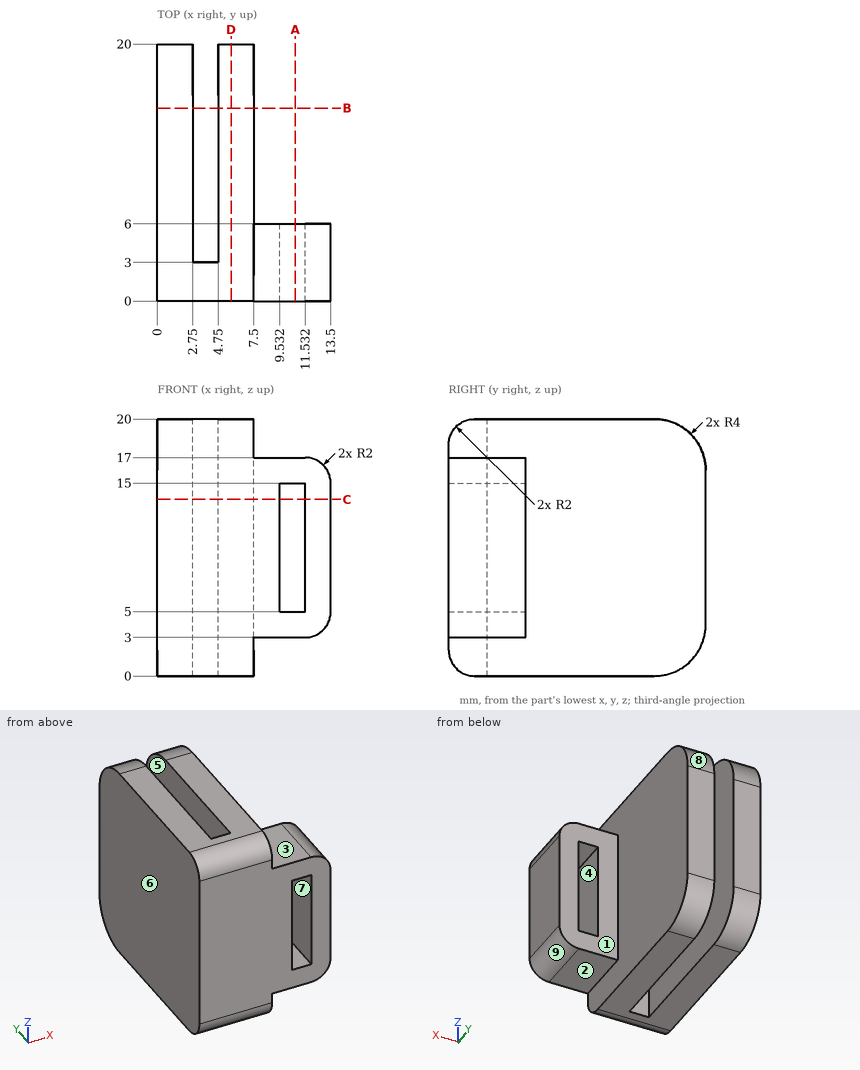
Verification items for this drawing (mm, ordinates from the low corner). A direction names the side the tool comes from. Give positions to 0.01 mm unless a question says otherwise; leave off trailing zeros. Write each loop counter-clockwise with the first axis right and the second up, starting at its lowest first coordinate (ties: lowest second). Pieces come first, ordered by that corner, then holes. Notation, with made-up numbers: (78.5, -20.75) -> (122.5, -20.75) arc R27 ccw to (122.5, 5.25) -> close; hole circle Ø2 at (24.5, 20). An arc over 180 degrees is marked (long way). Use CSV: the item, a comma, the result in double quotes.
(1) Sectioned sample at B-B (y = 15). Record the cut outline in (x, z), plus the area to 3 significant figures.
Derived:
outline,"(0, 0) -> (2.75, 0) -> (2.75, 20) -> (0, 20) -> close; (4.75, 0) -> (7.5, 0) -> (7.5, 20) -> (4.75, 20) -> close"
area,"110 mm^2"
(2) Material ranges on L1, parallel to X at y = 4.5, z = 12.25; L2, parallel to X at y = 16.5, z = 15.25; L3, parallel to Z at x = 10.5, y = 3.5, recorded low to high.
Derived:
L1,"x = 0 to 2.75, 4.75 to 9.53, 11.53 to 13.5"
L2,"x = 0 to 2.75, 4.75 to 7.5"
L3,"z = 3 to 5, 15 to 17"
(3) Set-up check for the marked faces 1, 2, 3, 4 and 5: record each of +Z, -Z, +X, -X, +Y, -Y from which the full face is reachable in a straight line by a thin tool's end or side.
Derived:
face 1,"+Z, -Z, +X, +Y"
face 2,"-Z, +X, +Y, -Y"
face 3,"+Z, +X, +Y, -Y"
face 4,"+Y, -Y"
face 5,"+Z, -Z, +Y"
(4) Sectioned sample at D-D (x = 5.75). Record the cut outline in (y, z), plus the area to 3 significant figures.
Derived:
outline,"(0, 2) arc R2 ccw to (2, 0) -> (16, 0) arc R4 ccw to (20, 4) -> (20, 16) arc R4 ccw to (16, 20) -> (2, 20) arc R2 ccw to (0, 18) -> close"
area,"391 mm^2"
(5) Sectioned sample at A-A (x = 10.75). Record the cut outline in (y, z).
Derived:
outline,"(0, 3) -> (6, 3) -> (6, 5) -> (0, 5) -> close; (0, 15) -> (6, 15) -> (6, 17) -> (0, 17) -> close"
(6) Sectioned sample at C-C (z = 13.75). Record the cut outline in (x, y).
Derived:
outline,"(0, 0) -> (9.53, 0) -> (9.53, 6) -> (7.5, 6) -> (7.5, 20) -> (4.75, 20) -> (4.75, 3) -> (2.75, 3) -> (2.75, 20) -> (0, 20) -> close; (11.53, 0) -> (13.5, 0) -> (13.5, 6) -> (11.53, 6) -> close"
(7) Go/stop test with flat-tipped pins: pin 1 (1.6 mm diameter, centred on x = 11, y = 3.5, fed in from +Z); pin 2 (5 mm diameter, centred on y = 14.5, z = 9, fed in from +X); pin 3 (4.5 mm diameter, centred on x = 10, y = 3.5, fed in from -Z); pin 4 (2 mm diameter, centred on x = 4, y = 8, fed in from -Z). Record where each tip stops, or that it passes through.
Derived:
pin 1,"stops at z = 17"
pin 2,"stops at x = 7.5"
pin 3,"stops at z = 3"
pin 4,"stops at z = 0"
(8) Release check for a two-part mould opening along X. For the marked faces 6, 7, 8 and 9 record: +X half, -X half, draft (parallel to the pull), parting line (faces both ways), or undercut.
Derived:
face 6,"-X half"
face 7,"undercut"
face 8,"draft"
face 9,"+X half"
